Geometry: final body of the model. Coordinates: model frame, mm. A direction names the side the tool comes from. Round coordinates to 2 decimals unless told otherwise and drop trailing zeros. Loops run counter-clockwise (first coordinate to the right, second up) from the corner with the lowest first, then second, coordinate; pieces in that order, holes last. Notation, with made-up numbers: (74, 16.25) - (99, 16.25) arc R12 ccw to (99, 29.25) - close; hole circle Ø6 at (84, 61.5). An arc over 180 degrees is marked (long way). Use CSV: the item, a comma, the result in double quotes.
Autodesk Inventor part; units mm, degrees
ref_plane "YZ Plane" through (0, 0, 0) normal (1, 0, 0) x (0, 1, 0)
ref_plane "XZ Plane" through (0, 0, 0) normal (0, 1, 0) x (-1, 0, 0)
ref_plane "XY Plane" through (0, 0, 0) normal (0, 0, 1) x (1, 0, 0)
sketch "Boceto1" plane through (0, 0, 0) normal (0, 0, 1) x (1, 0, 0)
  circle A0 centre (0, 0) radius 6
  dimension "d0" = 12
extrude "Extrusión1" add sketch "Boceto1" along normal blind 6
sketch "Boceto2" plane through (0, 0, 6) normal (0, 0, 1) x (1, 0, 0)
  circle A0 centre (0, 0) radius 10
  dimension "d3" = 20
extrude "Extrusión2" add sketch "Boceto2" along normal blind 4
sketch "Boceto3" plane through (0, 0, 0) normal (0, 0, -1) x (-1, 0, 0)
  line L0 (0, 3.4641) -> (3, 1.7321)
  line L1 (3, 1.7321) -> (3, -1.7321)
  line L2 (3, -1.7321) -> (0, -3.4641)
  line L3 (0, -3.4641) -> (-3, -1.7321)
  line L4 (-3, -1.7321) -> (-3, 1.7321)
  line L5 (-3, 1.7321) -> (0, 3.4641)
  point P0 (0, 0)
  point P1 (0, 0)
  point P2 (3, 0)
  dimension "d6" = 6
extrude "Extrusión3" cut sketch "Boceto3" against normal through all
properties part number "SoporteEje"
Item 1: Section C-C on x = 0.25. Return the cut outline in (y, z).
Final values:
outline,"(-10, 6) - (-5.99, 6) - (-5.99, 0) - (-3.32, 0) - (-3.32, 10) - (-10, 10) - close; (3.32, 0) - (5.99, 0) - (5.99, 6) - (10, 6) - (10, 10) - (3.32, 10) - close"
Item 2: Section B-B on z = 4.5. Return the cut outline in (x, y).
Final values:
outline,"circle Ø12 at (0, 0); hole (-3, -1.73) - (0, -3.46) - (3, -1.73) - (3, 1.73) - (0, 3.46) - (-3, 1.73) - close"
Item 3: Section A-A on y = 0. Return the cut outline in (x, z), plus the area to 3 significant figures.
Final values:
outline,"(-10, 6) - (-6, 6) - (-6, 0) - (-3, 0) - (-3, 10) - (-10, 10) - close; (3, 0) - (6, 0) - (6, 6) - (10, 6) - (10, 10) - (3, 10) - close"
area,"92.0 mm²"
Item 4: Pin query (flat end, axial travel): P1, Ø1.7, axis at y = 0, z = 2.5, coming from the +X side; P2, Ø1.5, axis at x = -4.5, z = 5, coming from the -Y side; P3, Ø1.5, axis at x = 5, z = 4.5, coming from the +Y side; P4, Ø1, axis at y = 0.5, z = 7, coming from the -X side. Return the tip coordinate at first contact, or that it passes through.
Final values:
P1,"stops at x = 6"
P2,"stops at y = -4.68"
P3,"stops at y = 4.24"
P4,"stops at x = -10"
Item 5: Reachability of faces 1 (the flat face through (-3, 0, 5)), 2 (the flat face through (-2.4, 2.4, 10)), 3 (the flat face through (7, 0, 6)) from +Z, -Z, +X, -X, +Y, -Y: full face, straight path, thin tool, end or side. Return the list, or none.
Final values:
face 1,"+Z, -Z"
face 2,"+Z, +X, -X, +Y, -Y"
face 3,"-Z"
Item 6: Section D-D on y = 3.75. Return the cut outline in (x, z), plus the area to 3 significant figures.
Final values:
outline,"(-9.27, 6) - (-4.68, 6) - (-4.68, 0) - (4.68, 0) - (4.68, 6) - (9.27, 6) - (9.27, 10) - (-9.27, 10) - close"
area,"130 mm²"
Item 7: Mould query, pull axis X, two halves, no side actions, for faces 4 (the flat face through (-1.5, 2.6, 4.9)), 5 (the flat face through (3, -3, 0)), 6 (the cylindrical face through (-6, 0, 3)), 7 (the flat face through (-1.5, -2.6, 4.9)). Classes: released by +X, released by -X, zero draft, split by the parting line, or undercut.
Final values:
face 4,"undercut"
face 5,"zero draft"
face 6,"split by the parting line"
face 7,"undercut"
Item 8: Material intervals for line 1 (Y direction, x = 8, z = 7.75); line 2 (Z direction, x = 6.25, y = -3.5); line 3 (X direction, y = 2, z = 4.75), sorted ascending.
Final values:
line 1,"y = -6 to 6"
line 2,"z = 6 to 10"
line 3,"x = -5.66 to -2.54, 2.54 to 5.66"
